CAD build for the part. Positions are in the model's coordinates, mm. A direction names the side the tool comes from. Round coordinates to 2 decimals unless told otherwise and drop trailing zeros. Loops run counter-clockwise (first coordinate to the right, second up) from the corner with the lowest first, then second, coordinate; pieces in that order, holes last. Notation, with made-up numbers: (-35.75, -29) - (18.25, -29) arc R15 ccw to (18.25, -20) - close; hole circle Ø2 at (76.25, -3). An arc over 180 degrees is marked (long way). Use one line per item in the form item = value.
from build123d import *

# Parameters (mm, degrees)
F1_DEPTH      = 150
F1_DEPTH_BACK = 150


with BuildPart() as f1:
    # F0 (on Front) → F1 (new body, two sides)
    with BuildSketch(Plane.XZ) as f1_sk:
        Polygon((-75, 25), (-75, -25), (75, -25), (75, 25), (64.2, 25), (64.2, 18), (68, 18), (68, 10), (52, 10), (52, 18), (55.8, 18), (55.8, 25), (4.2, 25), (4.2, 18), (8, 18), (8, 10), (-8, 10), (-8, 18), (-4.2, 18), (-4.2, 25), (-55.8, 25), (-55.8, 18), (-52, 18), (-52, 10), (-68, 10), (-68, 18), (-64.2, 18), (-64.2, 25), align=None)
    extrude(amount=-F1_DEPTH)
    extrude(f1_sk.sketch, amount=F1_DEPTH_BACK)


solid = f1.part
1) Two-plate mould, pull along X, no slides. Class faces 1 (the flat face through (75, 2, 0)), 2 (the flat face through (64.2, 2, 22)), 3 (the flat face through (-55.8, 2, 22)), 4 (the flat face through (70, 2, 25)): +X half, -X half, draft (parallel to the pull), parting line (faces both ways), or undercut.
Report:
face_1 = +X half
face_2 = undercut
face_3 = undercut
face_4 = draft
2) Drill centre lines: probe 1 along X at (y, z) = (126.5, 13.5); probe 2 along Z at (x, y) = (-5, -1); probe 3 along Z at (x, y) = (59.5, 62). Where is each one in solid material? Low to high.
Report:
probe_1 = -75 to -68, -52 to -8, 8 to 52, 68 to 75
probe_2 = -25 to 10, 18 to 25
probe_3 = -25 to 10
3) Slice it at B-B (y = -27.5). Write the cut outline in (x, z).
Report:
outline = (-75, -25) - (75, -25) - (75, 25) - (64.2, 25) - (64.2, 18) - (68, 18) - (68, 10) - (52, 10) - (52, 18) - (55.8, 18) - (55.8, 25) - (4.2, 25) - (4.2, 18) - (8, 18) - (8, 10) - (-8, 10) - (-8, 18) - (-4.2, 18) - (-4.2, 25) - (-55.8, 25) - (-55.8, 18) - (-52, 18) - (-52, 10) - (-68, 10) - (-68, 18) - (-64.2, 18) - (-64.2, 25) - (-75, 25) - close
4) Slice it at C-C (x = -60.5). Write the cut outline in (y, z), plus the area to 3 significant figures.
Report:
outline = (-150, -25) - (150, -25) - (150, 10) - (-150, 10) - close
area = 10,500 mm^2
5) Tool access for faces 5 (the flat face through (-75, 2, 0)), 6 (the flat face through (-4.2, 2, 21)), 7 (the flat face through (-68, 2, 14)): list every direction of +Z, -Z, +X, -X, +Y, -Y with a clear straight run to the whole face (end or side of a thin tool).
Report:
face_5 = +Z, -Z, -X, +Y, -Y
face_6 = +Z, +Y, -Y
face_7 = +Y, -Y
6) Slice it at A-A (z = 13). Write the cut outline in (x, y), plus the area to 3 significant figures.
Report:
outline = (-75, -150) - (-68, -150) - (-68, 150) - (-75, 150) - close; (-52, -150) - (-8, -150) - (-8, 150) - (-52, 150) - close; (8, -150) - (52, -150) - (52, 150) - (8, 150) - close; (68, -150) - (75, -150) - (75, 150) - (68, 150) - close
area = 30,600 mm^2
